Here's the drawing with two shaded views (mm, measured from the low corner). I have some questions. A direction names the side the tool comes from. Give positions to 0.01 mm unless a question says otherwise; leave off trailing zeros. Order: outer loops, then holes, each group sorted by start corner. A loop starts at its lowest first (then second) coordinate and runs counter-clockwise, first axis right, second up. Notation, with made-up numbers: M -19.75,55.25 L -6.75,55.25 A18 cw -6.75,72.25 Z; hole C -20.75,21.25 d8. An arc over 180 degrees is marked long. Write each question's results on one line, items separated by ' | '.
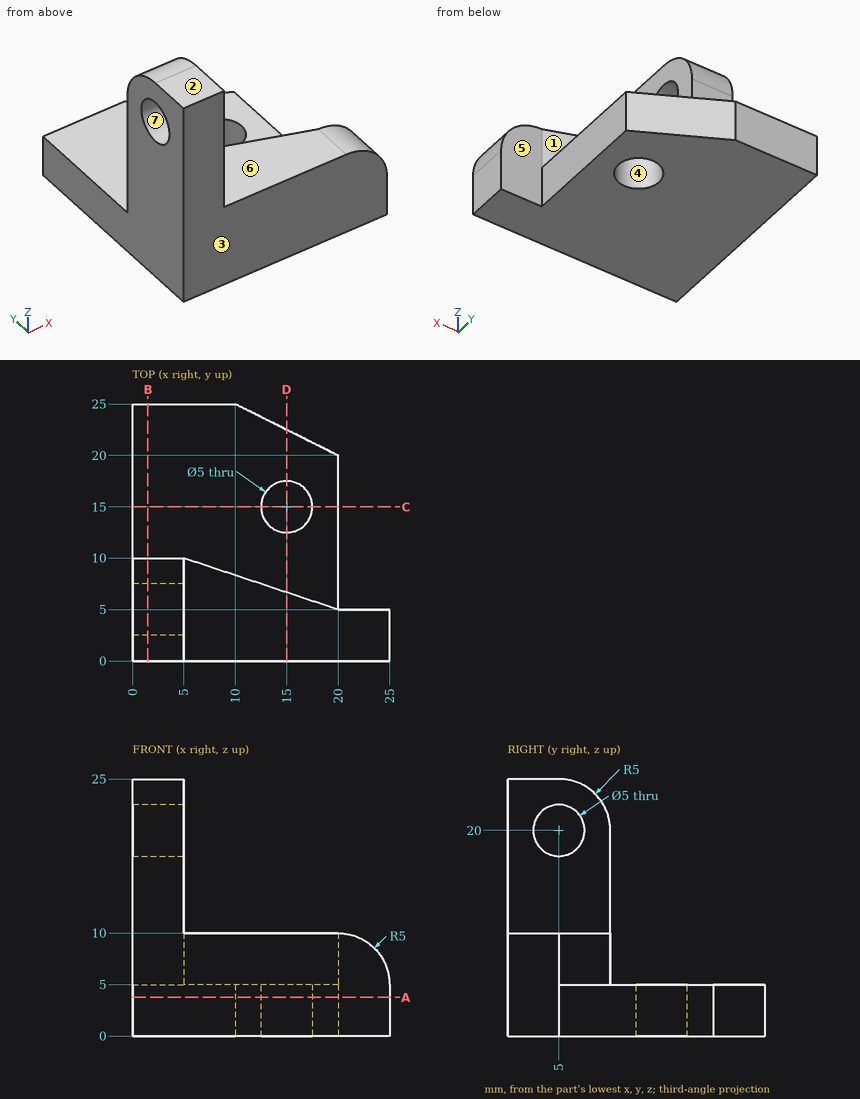
(1) I need wall thicknesses on L1, parallel to Y at x = 15, z = 1.5; L2, parallel to X at y = 2.25, z = 17.75; L3, parallel to Y at x = 2.75, z = 20. Which ranges of each line are inside material? Lowest first, please. Write a range as from..to.
Data:
L1: y = 0..12.5, 17.5..22.5 | L2: x = 0..5 | L3: y = 0..2.5, 7.5..10
(2) Will these pins go through, and if not, where does the flat tip stop? P1, Ø2.5, axis at x = 21.5, z = 2.5, coming from the +Y side; P2, Ø5.5, axis at x = 2.5, z = 12.5, coming from the +Y side; P3, Ø2.5, axis at y = 11, z = 1.5, coming from the +X side.
Data:
P1: stops at y = 5 | P2: stops at y = 10 | P3: stops at x = 20
(3) Imagine slicing it at B-B, the plane x = 1.5. Write out the boundary of the cut face in (y, z), plus the area to 3 significant figures.
Data:
outline: M 0,0 L 25,0 L 25,5 L 10,5 L 10,20 A5 ccw 5,25 L 0,25 Z; hole C 5,20 d5 | area: 300 mm2
(4) We'd pull the mould along Y, two halves only. Please class the marked faces 1, 2, 3 and 4: +Y half, -Y half, draft (parallel to the pull), parting line (faces both ways), or undercut.
Data:
face 1: +Y half | face 2: draft | face 3: -Y half | face 4: undercut
(5) For the marked faces 5, 6 and 7, which set-ups out of +Z, -Z, +X, -X, +Y, -Y let a thin tool reach every point of the face, with its end or its side?
Data:
face 5: +Z, -Z, +X, +Y | face 6: +Z, +X, +Y, -Y | face 7: +X, -X
(6) Imagine slicing it at C-C, the plane y = 15. Write out the boundary of the cut face in (x, z), plus the area to 3 significant figures.
Data:
outline: M 0,0 L 12.5,0 L 12.5,5 L 0,5 Z; M 17.5,0 L 20,0 L 20,5 L 17.5,5 Z | area: 75.0 mm2
(7) Imagine slicing it at A-A, the plane z = 3.75. Write out the boundary of the cut face in (x, y).
Data:
outline: M 0,0 L 25,0 L 25,5 L 20,5 L 20,20 L 10,25 L 0,25 Z; hole C 15,15 d5
(8) Imagine slicing it at D-D, the plane x = 15. Write out the boundary of the cut face in (y, z), plus the area to 3 significant figures.
Data:
outline: M 0,0 L 12.5,0 L 12.5,5 L 6.67,5 L 6.67,10 L 0,10 Z; M 17.5,0 L 22.5,0 L 22.5,5 L 17.5,5 Z | area: 121 mm2
